from build123d import *

# Parameters (mm, degrees)
F2_R     = 1.65
F3_DEPTH = 10.001
F5_DEPTH = 2
F7_DEPTH = 10.001
F9_DEPTH = 2


# Not quite as in the source:
# - ends of sketch curves that miss each other by under 0.0002 mm in the source are joined


with BuildPart() as f1:
    # F0 (on Front) → F1 (revolve)
    with BuildSketch(Plane.XZ):
        Polygon((20.5, 16.3456536829), (20.5, 8.3456536829), (23, 8.3456536829), (23, 10.3456536829), (21.5, 10.3456536829), (21.5, 12.8456536829), (23, 12.8456536829), (23, 18.3456536829), (14.75, 18.3456536829), (14.75, 16.3456536829), align=None)
    revolve(axis=Axis((0, 0, 17.3456536829), (0, 0, -1)))

    # F2 (on face) → F3 (cut, through all)
    with BuildSketch(Plane.XY.offset(18.3456536829)):
        with Locations((0, 17)):
            Circle(F2_R)
        with Locations((17, 0)):
            Circle(F2_R)
        with Locations((-17, 0)):
            Circle(F2_R)
        with Locations((0, -17)):
            Circle(F2_R)
    extrude(amount=-F3_DEPTH, mode=Mode.SUBTRACT)

    # F4 (on face) → F5 (join)
    with BuildSketch(Plane.XY.offset(18.3456536829)):
        with BuildLine():
            Line((-1.6499559837, 14.6574262833), (-1.6499626499, 9.8629419168))
            ThreePointArc((-1.6499626499, 9.8629419168), (-7.0714247823, 7.0707108234), (-9.8631084617, 1.6489667897))
            Line((-9.8631084617, 1.6489667897), (-14.6575583453, 1.6487823851))
            ThreePointArc((-14.6575583453, 1.6487823851), (-14.7499999873, -0.0006126499), (-14.6574213285, -1.6499999999))
            Line((-14.6574213285, -1.6499999999), (-9.8629356685, -1.6499999997))
            ThreePointArc((-9.8629356685, -1.6499999997), (-7.0710642548, -7.071071369), (-1.6499900767, -9.8629373285))
            Line((-1.6499900767, -9.8629373285), (-1.6499967429, -14.6574216951))
            ThreePointArc((-1.6499967429, -14.6574216951), (0, -14.75), (1.6499967429, -14.6574216951))
            Line((1.6499967429, -14.6574216951), (1.6499900767, -9.8629373285))
            ThreePointArc((1.6499900767, -9.8629373285), (7.071064255, -7.0710713687), (9.8629356686, -1.649999999))
            Line((9.8629356686, -1.649999999), (14.6574213286, -1.6499999989))
            ThreePointArc((14.6574213286, -1.6499999989), (14.7268371451, -0.8262975866), (14.75, 0))
            ThreePointArc((14.75, 0), (14.7268396846, 0.8262523244), (14.6574314707, 1.6499099011))
            Line((14.6574314707, 1.6499099011), (9.862981587, 1.6497254965))
            ThreePointArc((9.862981587, 1.6497254965), (7.0711528227, 7.0709828), (1.6499626499, 9.8629419168))
            Line((1.6499626499, 9.8629419168), (1.6499559837, 14.6574262833))
            ThreePointArc((1.6499559837, 14.6574262833), (0, 14.75), (-1.6499559837, 14.6574262833))
        make_face()
        with BuildLine():
            Line((-1.649952744, 16.9875123006), (-1.6499559837, 14.6574262833))
            ThreePointArc((-1.6499559837, 14.6574262833), (0, 14.75), (1.6499559837, 14.6574262833))
            Line((1.6499559837, 14.6574262833), (1.649952744, 16.9875123006))
            ThreePointArc((1.649952744, 16.9875123006), (0, 15.35), (-1.649952744, 16.9875123006))
        make_face()
        with BuildLine():
            Line((16.9999365375, 1.6499999988), (14.6574314707, 1.6499099011))
            ThreePointArc((14.6574314707, 1.6499099011), (14.7268396846, 0.8262523244), (14.75, 0))
            ThreePointArc((14.75, 0), (14.7268371451, -0.8262975866), (14.6574213286, -1.6499999989))
            Line((14.6574213286, -1.6499999989), (16.9999365375, -1.6499999988))
            ThreePointArc((16.9999365375, -1.6499999988), (15.35, 0), (16.9999365375, 1.6499999988))
        make_face()
        with BuildLine():
            ThreePointArc((-14.6574213285, -1.6499999999), (-14.7499999873, -0.0006126499), (-14.6575583453, 1.6487823851))
            Line((-14.6575583453, 1.6487823851), (-16.9343843655, 1.6486948136))
            ThreePointArc((-16.9343843655, 1.6486948136), (-15.8103013413, 1.1432922205), (-15.35, 0))
            ThreePointArc((-15.35, 0), (-15.833273811, -1.166726189), (-17, -1.65))
            Line((-17, -1.65), (-14.6574213285, -1.6499999999))
        make_face()
        with BuildLine():
            ThreePointArc((1.6499967429, -14.6574216951), (0, -14.75), (-1.6499967429, -14.6574216951))
            Line((-1.6499967429, -14.6574216951), (-1.65, -16.9999977059))
            ThreePointArc((-1.65, -16.9999977059), (1.1471e-06, -15.35), (1.65, -17))
            Line((1.65, -17), (1.6499967429, -14.6574216951))
        make_face()
    extrude(amount=-F5_DEPTH)

    # F6 (on face) → F7 (cut, through all)
    with BuildSketch(Plane.XY.offset(18.3456536829)):
        with BuildLine():
            ThreePointArc((-1.8447082725, 14.6341911765), (-2.634985421, 15.5658271264), (-2.9882989803, 16.7352941176))
            ThreePointArc((-2.9882989803, 16.7352941176), (-12.0208152802, 12.0208152802), (-16.7352941176, 2.9882989803))
            ThreePointArc((-16.7352941176, 2.9882989803), (-15.5658271264, 2.634985421), (-14.6341911765, 1.8447082725))
            ThreePointArc((-14.6341911765, 1.8447082725), (-10.4298250225, 10.4298250225), (-1.8447082725, 14.6341911765))
        make_face()
        with BuildLine():
            ThreePointArc((2.9882989803, 16.7352941176), (2.634985421, 15.5658271264), (1.8447082725, 14.6341911765))
            ThreePointArc((1.8447082725, 14.6341911765), (10.4298250225, 10.4298250225), (14.6341911765, 1.8447082725))
            ThreePointArc((14.6341911765, 1.8447082725), (15.5658271264, 2.634985421), (16.7352941176, 2.9882989803))
            ThreePointArc((16.7352941176, 2.9882989803), (12.0208152802, 12.0208152802), (2.9882989803, 16.7352941176))
        make_face()
        with BuildLine():
            ThreePointArc((16.7352941176, -2.9882989803), (15.5658271264, -2.634985421), (14.6341911765, -1.8447082725))
            ThreePointArc((14.6341911765, -1.8447082725), (10.4298250225, -10.4298250225), (1.8447082725, -14.6341911765))
            ThreePointArc((1.8447082725, -14.6341911765), (2.634985421, -15.5658271264), (2.9882989803, -16.7352941176))
            ThreePointArc((2.9882989803, -16.7352941176), (12.0208152802, -12.0208152802), (16.7352941176, -2.9882989803))
        make_face()
        with BuildLine():
            ThreePointArc((-1.8447082725, -14.6341911765), (-10.4298250225, -10.4298250225), (-14.6341911765, -1.8447082725))
            ThreePointArc((-14.6341911765, -1.8447082725), (-15.5658271264, -2.634985421), (-16.7352941176, -2.9882989803))
            ThreePointArc((-16.7352941176, -2.9882989803), (-12.0208152802, -12.0208152802), (-2.9882989803, -16.7352941176))
            ThreePointArc((-2.9882989803, -16.7352941176), (-2.634985421, -15.5658271264), (-1.8447082725, -14.6341911765))
        make_face()
        Polygon((0.0182914075, -7.1591199709), (6.2091254673, -3.5637191619), (6.1908340598, 3.595400809), (-0.0182914075, 7.1591199709), (-6.2091254673, 3.5637191619), (-6.1908340598, -3.595400809), align=None)
    extrude(amount=-F7_DEPTH, mode=Mode.SUBTRACT)

    # F8 (on face) → F9 (join)
    with BuildSketch(Plane(origin=(0, 0, 16.3456536829), x_dir=(1, 0, 0), z_dir=(0, 0, -1))):
        with BuildLine():
            ThreePointArc((9.862981587, -1.6497254965), (9.965686526, -0.8277028844), (10, 0))
            ThreePointArc((10, 0), (9.9656750069, 0.8278415651), (9.8629356686, 1.649999999))
            ThreePointArc((9.8629356686, 1.649999999), (7.071064255, 7.0710713687), (1.6499900767, 9.8629373285))
            ThreePointArc((1.6499900767, 9.8629373285), (0, 10), (-1.6499900767, 9.8629373285))
            ThreePointArc((-1.6499900767, 9.8629373285), (-7.0710642548, 7.071071369), (-9.8629356685, 1.6499999997))
            ThreePointArc((-9.8629356685, 1.6499999997), (-9.9999999863, 0.0005237796), (-9.8631084617, -1.6489667897))
            ThreePointArc((-9.8631084617, -1.6489667897), (-7.0714247823, -7.0707108234), (-1.6499626499, -9.8629419168))
            ThreePointArc((-1.6499626499, -9.8629419168), (0, -10), (1.6499626499, -9.8629419168))
            ThreePointArc((1.6499626499, -9.8629419168), (7.0711528227, -7.0709828), (9.862981587, -1.6497254965))
        make_face()
        Polygon((-6.1908340598, 3.595400809), (0.0182914075, 7.1591199709), (6.2091254673, 3.5637191619), (6.1908340598, -3.595400809), (-0.0182914075, -7.1591199709), (-6.2091254673, -3.5637191619), align=None, mode=Mode.SUBTRACT)
    extrude(amount=F9_DEPTH)


solid = f1.part
Model file for the job. Use its own axes, mm. A direction names the side the tool comes from. Give positions to 0.01 mm unless a question says otherwise; leave off trailing zeros. Loops run counter-clockwise (first coordinate to the right, second up) from the corner with the lowest first, then second, coordinate; pieces in that order, holes last. Notation, with made-up numbers: (19.25, 35) - (77.25, 35) arc R25 cw to (77.25, 47) - close; hole circle Ø3 at (-21.75, 35). An arc over 180 degrees is marked (long way). Use one line per item in the form item = value.
(1) Cut at B-B (y = -8.5). Give the cut face in (x, z), then the cut area to 3 significant figures.
Determined:
outline = (-21.37, 8.35) - (-18.65, 8.35) - (-18.65, 16.35) - (-14.72, 16.35) - (-14.72, 18.35) - (-21.37, 18.35) - (-21.37, 12.85) - (-19.75, 12.85) - (-19.75, 10.35) - (-21.37, 10.35) - close; (-5.27, 14.35) - (5.27, 14.35) - (5.27, 18.35) - (-5.27, 18.35) - close; (14.72, 16.35) - (18.65, 16.35) - (18.65, 8.35) - (21.37, 8.35) - (21.37, 10.35) - (19.75, 10.35) - (19.75, 12.85) - (21.37, 12.85) - (21.37, 18.35) - (14.72, 18.35) - close
area = 104 mm^2
(2) Pull direction Z, two halves, no side cores. Call faces 4 (the face through (-2.799, -21.317, 11.613)), 5 (the face through (0, -11, 16.346)), 6 (the face through (-11.92, 12.12, 17.36)): pulls with the +Z half, pulls with the -Z half, needs draft (parallel to the pull), parting line crosses it, or undercut.
Determined:
face_4 = undercut
face_5 = pulls with the -Z half
face_6 = needs draft
(3) Cut at A-A (z = 15). Give the cut face in (x, y), then the cut area to 3 significant figures.
Determined:
outline = circle Ø46 at (0, 0); circle Ø20 at (0, 0); hole circle Ø41 at (0, 0); hole (-6.21, 3.56) - (-6.19, -3.6) - (0.02, -7.16) - (6.21, -3.56) - (6.19, 3.6) - (-0.02, 7.16) - close
area = 523 mm^2
(4) Drill centre lines: L1, parallel to Y at x = 0, z = 17.4; L2, parallel to X at y = 0, z = 16.9; L3, parallel to Y at x = 0, z = 13.5. Where is each one in solid material? Low to high.
Determined:
L1 = -23 to -18.65, -15.35 to -7.15, 7.15 to 15.35, 18.65 to 23
L2 = -23 to -18.65, -15.35 to -6.2, 6.2 to 15.35, 18.65 to 23
L3 = -23 to -20.5, 20.5 to 23
(5) Drop flat-ended pins along their axis: P1, Ø3, axis at y = 17.5, z = 14.5, coming from the +X side; P2, Ø0.6, axis at y = -12.5, z = 17.5, coming from the -X side; P3, Ø2, axis at x = -17.5, z = 16.5, coming from the -Y side; P4, Ø6, axis at x = -2.5, y = -0.5, coming from the -Z side. Give the stop position or say it passes through.
Determined:
P1 = 16.52
P2 = -19.5
P3 = -16.02
P4 = through
(6) Cut at C-C (y = 6.5). Give the cut face in (x, z), then the cut area to 3 significant figures.
Determined:
outline = (-22.06, 8.35) - (-19.44, 8.35) - (-19.44, 16.35) - (-15.71, 16.35) - (-15.71, 18.35) - (-22.06, 18.35) - (-22.06, 12.85) - (-20.49, 12.85) - (-20.49, 10.35) - (-22.06, 10.35) - close; (-7.6, 14.35) - (-1.15, 14.35) - (-1.15, 18.35) - (-7.6, 18.35) - close; (1.13, 14.35) - (7.6, 14.35) - (7.6, 18.35) - (1.13, 18.35) - close; (15.71, 16.35) - (19.44, 16.35) - (19.44, 8.35) - (22.06, 8.35) - (22.06, 10.35) - (20.49, 10.35) - (20.49, 12.85) - (22.06, 12.85) - (22.06, 18.35) - (15.71, 18.35) - close
area = 111 mm^2
(7) 3-axis set-ups, long thin cutter, end or side, ignore diameter. For faces 1 (the face through (-12.12, -11.92, 17.36)), 2 (the face through (17, 14, 10.346)), 3 (the face through (21, 2, 8.346)): which of +Z, -Z, +X, -X, +Y, -Y reach the whole face in a straight line?
Determined:
face_1 = +Z, -Z
face_2 = none
face_3 = -Z, +X, -X, +Y, -Y
